Print and shaded views of the part. All mm, measured from the part's lowest x, y and z. A direction names the side the tool comes from. Round coordinates to 2 decimals unless told otherwise and drop trailing zeros. Write each loop counter-clockwise with the first axis right and the second up, starting at its lowest first coordinate (ties: lowest second). Pieces come first, ordered by that corner, then holes. Notation, with made-up numbers: (-16, 79.5) -> (14, 79.5) arc R24 ccw to (14, 102.5) -> close; hole circle Ø2 at (2.25, 68). An arc over 180 degrees is marked (long way). Use CSV: the item, a comma, the result in double quotes. Start each with the question number.
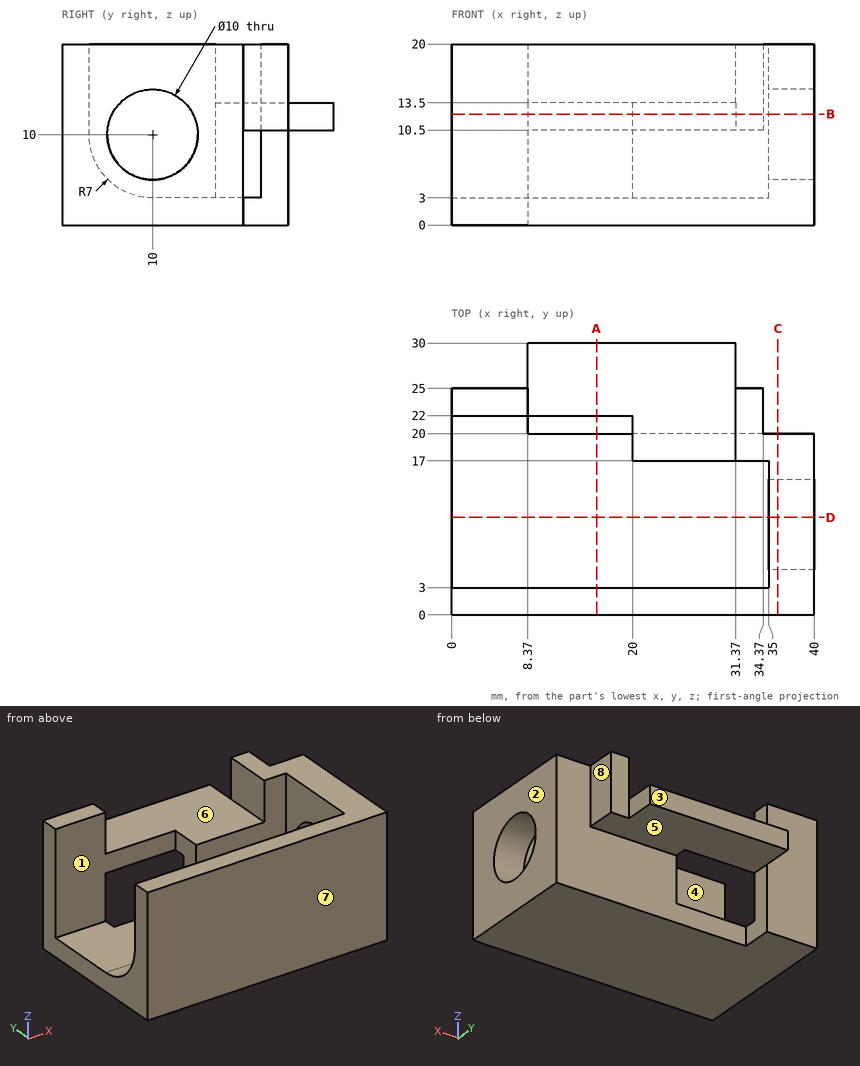
1. Pull direction Y, two halves, no side cores. Call the marked faces 1, 2 and 3: released by +Y, released by -Y, zero draft, split by the parting line, or undercut.
2. Flat gauge pins, fed straight in: pin 1 (2 mm diameter, centred on y = 13.5, z = 6.5, fed in from -X); pin 2 (3 mm diameter, centred on x = 26.5, y = 27.5, fed in from -Z); pin 3 (6 mm diameter, centred on x = 21, y = 16.5, fed in from +Z). Where does each tip first touch, or does it go through?
3. Band-saw the part on A-A (x = 16). List the corners of the cut face in (y, z).
4. Which spindle directions (+Z, -Z, +X, -X, +Y, -Y) get a long thin tool onto all of the face, cutting with end or side? Do the marked faces 4, 5, 6, 7 and 8. Say none if no direction does.
5. Band-saw the part on B-B (z = 12.25). List the corners of the cut face in (x, y) (1 decimal).
6. Band-saw the part on C-C (x = 36). List the corners of the cut face in (y, z).
7. Band-saw the part on D-D (y = 10.75). List the corners of the cut face in (x, z).
8. Drill centre lines: line 1 along Z through (x, y) = (38.85, 10); line 2 along Y through (x, z) = (4, 12). Where is each one in solid material? Low to high. Write a range as [from, to].
Answers below:
1,face 1,"undercut"
1,face 2,"zero draft"
1,face 3,"released by +Y"
2,pin 1,"stops at x = 35"
2,pin 2,"stops at z = 10.5"
2,pin 3,"stops at z = 13.5"
3,outline,"(0, 0) -> (20, 0) -> (20, 3) -> (10, 3) arc R7 cw to (3, 10) -> (3, 20) -> (0, 20) -> close; (22, 10.5) -> (30, 10.5) -> (30, 13.5) -> (22, 13.5) -> close"
4,face 4,"+Z, -X"
4,face 5,"-Z, +X, +Y"
4,face 6,"+Z, +Y"
4,face 7,"+Z, -Z, +X, -X, -Y"
4,face 8,"+Z, -Z, +X, +Y"
5,outline,"(0, 0) -> (40, 0) -> (40, 5.5) -> (35, 5.5) -> (35, 3) -> (0, 3) -> close; (0, 22) -> (20, 22) -> (20, 17) -> (35, 17) -> (35, 14.5) -> (40, 14.5) -> (40, 20) -> (34.4, 20) -> (34.4, 25) -> (31.4, 25) -> (31.4, 30) -> (8.4, 30) -> (8.4, 25) -> (0, 25) -> close"
6,outline,"(0, 0) -> (20, 0) -> (20, 20) -> (0, 20) -> close; hole circle Ø10 at (10, 10)"
7,outline,"(0, 0) -> (40, 0) -> (40, 5.06) -> (35, 5.06) -> (35, 3) -> (0, 3) -> close; (35, 14.94) -> (40, 14.94) -> (40, 20) -> (35, 20) -> close"
8,line 1,"z = [0, 5], [15, 20]"
8,line 2,"y = [0, 3], [22, 25]"
